from build123d import *

# Parameters (mm, degrees)
SKETCH1_W           = 5
SKETCH1_H           = 5
BOSS_EXTRUDE1_DEPTH = 110
SKETCH2_W           = 3
SKETCH2_H           = 3
CUT_EXTRUDE1_DEPTH  = 9
SKETCH3_W           = 3
SKETCH3_H           = 3
CUT_EXTRUDE2_DEPTH  = 9
SKETCH4_W           = 5
SKETCH4_H           = 5
BOSS_EXTRUDE2_DEPTH = 6
SKETCH5_R           = 1.4
BOSS_EXTRUDE3_DEPTH = 13


with BuildPart() as part:
    # Sketch1 → Boss-Extrude1 (new body)
    with BuildSketch(Plane.XY):
        with Locations((2.5, 2.5)):
            Rectangle(SKETCH1_W, SKETCH1_H)
    extrude(amount=BOSS_EXTRUDE1_DEPTH)

    # Sketch2 → Cut-Extrude1 (cut)
    with BuildSketch(Plane.ZY):
        with Locations((2.5, 2.5)):
            Rectangle(SKETCH2_W, SKETCH2_H)
        with Locations((107.5, 2.5)):
            Rectangle(SKETCH2_W, SKETCH2_H)
    extrude(amount=-CUT_EXTRUDE1_DEPTH, mode=Mode.SUBTRACT)

    # Sketch3 → Cut-Extrude2 (cut)
    with BuildSketch(Plane(origin=(0, 5, 0), x_dir=(1, 0, 0), z_dir=(0, 1, 0))):
        with Locations((2.5, -25.15)):
            Rectangle(SKETCH3_W, SKETCH3_H)
    extrude(amount=-CUT_EXTRUDE2_DEPTH, mode=Mode.SUBTRACT)

    # Sketch4 → Boss-Extrude2 (add)
    with BuildSketch(Plane(origin=(0, 0, 0), x_dir=(-1, 0, 0), z_dir=(0, -1, 0))):
        with Locations((-2.5, -70.15)):
            Rectangle(SKETCH4_W, SKETCH4_H)
    extrude(amount=BOSS_EXTRUDE2_DEPTH)

    # Sketch5 → Boss-Extrude3 (add)
    with BuildSketch(Plane.ZY):
        with Locations((70.15, -3)):
            Circle(SKETCH5_R)
    extrude(amount=-BOSS_EXTRUDE3_DEPTH)


solid = part.part
Can you work these out from the model? Positions are in its coordinate system, mm. A direction names the side the tool comes from. Give positions to 0.01 mm unless a question says otherwise; leave off trailing zeros. Order: outer loops, then holes, each group sorted by start corner. A loop starts at its lowest first (then second) coordinate and runs counter-clockwise, first axis right, second up. Notation, with made-up numbers: M 80.5,54 L 114.5,54 A11 ccw 114.5,70 Z; hole C 83.5,84 d8. An arc over 180 degrees is marked long. Use one line per item in the form item = value. Start each with the question number.
Item 1: If I drill on line 1 along Z through (x, y) = (3, -5.5); line 2 along X through (y, z) = (1.75, 63), over which ranges is the centre line in solid material (lowest first)?
Item 2: We'd pull the mould along X, two halves only. Please class faces 5 (the flat face through (2, 3, 26.65)), 6 (the flat face through (13, -3, 70)), 7 (the flat face through (3, -3, 72.65)): +X half, -X half, draft (parallel to the pull), parting line (faces both ways), or undercut.
Item 3: If we section it at B-B (x = 2.25): Write out the boundary of the cut face in (y, z).
Item 4: Will these pins go through, and if not, where does the flat tip stop? pin 1 Ø3.5 at (x, z) = (2, 108) entering from -Y; pin 2 Ø3.5 at (y, z) = (2.5, 25.5) entering from +X; pin 3 Ø3 at (x, y) = (9.5, 0.5) entering from +Z.
Item 5: If we section it at A-A (y = 2): Write out the boundary of the cut face in (x, z), then the cut area to 3 significant figures.
Item 6: If we section it at C-C (y = -3): Write out the boundary of the cut face in (x, z).
Item 7: If we section it at D-D (z = 70.15): Write out the boundary of the cut face in (x, y), then the cut area to 3 significant figures.
Item 8: For faces 1 (the flat face through (2, 3, 23.65)), 2 (the flat face through (2, 0, 33)), 3 (the flat face through (2, 2, 106)), 4 (the flat face through (2, 0, 91)), which set-ups out of +Z, -Z, +X, -X, +Y, -Y let a thin tool reach every point of the face, with its end or its side?
Outcome:
q1.line_1 = 67.65 to 72.65
q1.line_2 = 0 to 5
q2.face_5 = undercut
q2.face_6 = +X half
q2.face_7 = draft
q3.outline = M -6,67.65 L 0,67.65 L 0,26.65 L 5,26.65 L 5,110 L 0,110 L 0,72.65 L -6,72.65 Z; M 0,0 L 5,0 L 5,23.65 L 0,23.65 Z; hole M 1,1 L 4,1 L 4,4 L 1,4 Z; hole M 1,106 L 4,106 L 4,109 L 1,109 Z
q4.pin_1 = 0
q4.pin_2 = 5
q4.pin_3 = through
q5.outline = M 0,0 L 5,0 L 5,1 L 0,1 Z; M 0,4 L 5,4 L 5,106 L 0,106 Z; M 0,109 L 5,109 L 5,110 L 0,110 Z; hole M 1,23.65 L 4,23.65 L 4,26.65 L 1,26.65 Z
q5.area = 511 mm2
q6.outline = M 0,67.65 L 5,67.65 L 5,68.75 L 13,68.75 L 13,71.55 L 5,71.55 L 5,72.65 L 0,72.65 Z
q7.outline = M 0,-6 L 5,-6 L 5,-4.4 L 13,-4.4 L 13,-1.6 L 5,-1.6 L 5,5 L 0,5 Z
q7.area = 77.4 mm2
q8.face_1 = +Y, -Y
q8.face_2 = -Z, +X, -X, -Y
q8.face_3 = +X, -X
q8.face_4 = +Z, +X, -X, -Y
